Read the model definition and answer for the solid it produces. Units are mm, in the model's axes. Coordinates: 2 decimals unless noted, no trailing zeros. Order: outer loops, then holes, each group sorted by start corner. A loop starts at its lowest first (then second) coordinate and runs counter-clockwise, first axis right, second up. Notation, with made-up numbers: (-25, -35.75) -> (28, -35.75) arc R16 ccw to (28, -28.75) -> close; hole circle Ø6 at (85, 26.5). An arc over 180 degrees is marked (long way). Answer as a JSON object with one key per item and string values. Group by question number.
1) Section D-D on x = 6 is taken. Determine the outline of the cut face in (y, z), and give its area (3 significant figures).
2) Determine the mould class of faces 1 (the cylindrical face through (-21.55, 0.27, 23.496)), 2 (the cylindrical face through (25.489, 22.785, -0.28)), 3 (the cylindrical face through (-11.99, 0.53, -0.35)) for opening direction Y: released by +Y, released by -Y, zero draft, split by the parting line, or undercut.
3) Section A-A on y = 0 is taken. Determine the outline of the cut face in (x, z), and give its area (3 significant figures).
4) Section C-C on x = 0 is taken. Determine the outline of the cut face in (y, z).
5) Section B-B on z = -4 is taken. Determine the outline of the cut face in (x, y), and give its area (3 significant figures).
6) Consider L1, parallel to Y at x = 0, z = -11.5; L2, parallel to X at y = -0.5, z = 10.5; L3, parallel to Y at x = 2, z = 15.5. Determine where each line is inside the solid, lowest interval first.
from build123d import *

# Parameters (mm, degrees)
F0_W     = 49.890485
F0_H     = 48.57757
F0_R     = 12
F1_DEPTH = 25
F2_R     = 5


with BuildPart() as f1:
    # F0 (on Top) → F1 (new body, symmetric)
    with BuildSketch(Plane.XY):
        with Locations((1.969362, 0)):
            Rectangle(F0_W, F0_H)
        Circle(F0_R, mode=Mode.SUBTRACT)
    extrude(amount=F1_DEPTH, both=True)

    # F2
    f2_edges = [f1.edges().sort_by_distance(p)[0] for p in [
        (-22.97588, 24.288785, 0),
        (1.969363, 24.288785, 25),
        (-22.97588, 0, 25),
        (-22.97588, -24.288785, 0),
        (26.914605, 0, 25),
        (1.969363, -24.288785, 25),
        (26.914605, 24.288785, 0),
        (26.914605, -24.288785, 0),
        (26.914605, 0, -25),
        (1.969363, 24.288785, -25),
        (1.969363, -24.288785, -25),
    ]]
    fillet(f2_edges, radius=F2_R)


solid = f1.part
Worked answers:
{
 "1": {"outline": "(-24.29, -20) arc R5 ccw to (-19.29, -25) -> (-10.39, -25) -> (-10.39, 25) -> (-19.29, 25) arc R5 ccw to (-24.29, 20) -> close; (10.39, -25) -> (19.29, -25) arc R5 ccw to (24.29, -20) -> (24.29, 20) arc R5 ccw to (19.29, 25) -> (10.39, 25) -> close", "area": "1,370 mm²"},
 "2": {"face 1": "zero draft", "face 2": "released by +Y", "face 3": "undercut"},
 "3": {"outline": "(-22.98, -25) -> (-12, -25) -> (-12, 25) -> (-17.98, 25) arc R5 ccw to (-22.98, 20) -> close; (12, -25) -> (21.91, -25) arc R5 ccw to (26.91, -20) -> (26.91, 20) arc R5 ccw to (21.91, 25) -> (12, 25) -> close", "area": "1,280 mm²"},
 "4": {"outline": "(-24.29, -20) arc R5 ccw to (-19.29, -25) -> (-12, -25) -> (-12, 25) -> (-19.29, 25) arc R5 ccw to (-24.29, 20) -> close; (12, -25) -> (19.29, -25) arc R5 ccw to (24.29, -20) -> (24.29, 20) arc R5 ccw to (19.29, 25) -> (12, 25) -> close"},
 "5": {"outline": "(-22.98, -19.29) arc R5 ccw to (-17.98, -24.29) -> (21.91, -24.29) arc R5 ccw to (26.91, -19.29) -> (26.91, 19.29) arc R5 ccw to (21.91, 24.29) -> (-17.98, 24.29) arc R5 ccw to (-22.98, 19.29) -> close; hole circle Ø24 at (0, 0)", "area": "1,950 mm²"},
 "6": {"L1": "y = -24.29 to -12, 12 to 24.29", "L2": "x = -22.98 to -11.99, 11.99 to 26.91", "L3": "y = -24.29 to -11.83, 11.83 to 24.29"}
}
